The figure shows three views and two pictorial views of one solid part (mm, origin at its lowest corner). Answer the questions. A direction names the side the tool comes from. Coordinates: 2 decimals unless noted, no trailing zeros. Loops run counter-clockwise (first coordinate to the right, second up) from the corner with the lowest first, then second, coordinate; pieces in that order, holes last. Notation, with made-up numbers: M 10,13.25 L 18,13.25 A27 ccw 18,31.25 Z; hole C 3,54 d7. An arc over 180 degrees is marked long. Answer in a Markdown table with one row per item. Add a question column.
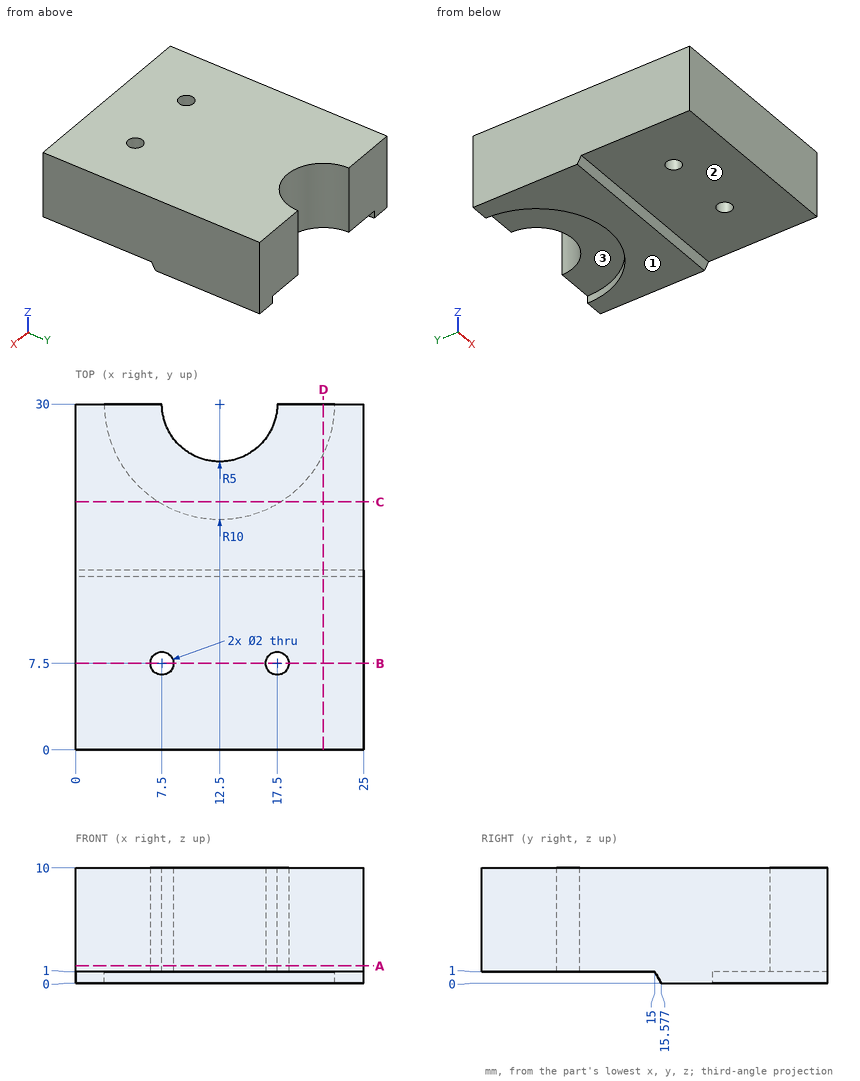
(1) For the marked faces 1, 2 and 3, determine the directions among +Z, -Z, +X, -X, +Y, -Y from which every point of the face is accessible in a straight line to the end or side of a thin tool.
(2) A cutting plane is placed at D-D (x = 21.5). Give the vertices of the cut face in (y, z).
(3) This flat-tipped pin is pushed along its axis until it touches: pin 1 (5 mm diameter, centred on x = 20.5, y = 5.5, fed in from -Z). Where does it stop, or does it pass through?
(4) A cutting plane is placed at A-A (z = 1.5). Give the vertices of the cut face in (x, y).
(5) Straight lines are drawn through the part: line 1 (X direction, y = 7.5, z = 6.5); line 2 (Z direction, x = 15.75, y = 11.5); line 3 (X direction, y = 26.25, z = 9.5) (1 decimal). For each, find the intervals that lie inside material, in ascending order.
(6) A cutting plane is placed at B-B (y = 7.5). Give the vertices of the cut face in (x, z).
(7) A cutting plane is placed at C-C (y = 21.5). Give the vertices of the cut face in (x, z).
Solved:
| question | item | result |
|---|---|---|
| 1 | face 1 | -Z, +X, -X, +Y, -Y |
| 1 | face 2 | -Z, +X, -X, -Y |
| 1 | face 3 | -Z, +Y |
| 2 | outline | M 0,1 L 15,1 L 15.58,0 L 25.64,0 L 25.64,1 L 30,1 L 30,10 L 0,10 Z |
| 3 | pin 1 | stops at z = 1 |
| 4 | outline | M 0,0 L 25,0 L 25,30 L 17.5,30 A5 cw 7.5,30 L 0,30 Z; hole C 7.5,7.5 d2; hole C 17.5,7.5 d2 |
| 5 | line 1 | x = 0 to 6.5, 8.5 to 16.5, 18.5 to 25 |
| 5 | line 2 | z = 1 to 10 |
| 5 | line 3 | x = 0 to 9.2, 15.8 to 25 |
| 6 | outline | M 0,1 L 6.5,1 L 6.5,10 L 0,10 Z; M 8.5,1 L 16.5,1 L 16.5,10 L 8.5,10 Z; M 18.5,1 L 25,1 L 25,10 L 18.5,10 Z |
| 7 | outline | M 0,0 L 7.23,0 L 7.23,1 L 17.77,1 L 17.77,0 L 25,0 L 25,10 L 0,10 Z |
